from build123d import *

# Parameters (mm, degrees)
BOSS_EXTRUDE1_DEPTH = 1
BOSS_EXTRUDE2_START = 1
BOSS_EXTRUDE2_DEPTH = 1
CUT_EXTRUDE1_REACH  = 128.037
CUT_EXTRUDE2_REACH  = 126.851
SKETCH4_R           = 1.25
CHAMFER1_SIZE       = 1.5
SKETCH5_W           = 55.9
SKETCH5_H           = 5
BOSS_EXTRUDE3_DEPTH = 1.5
CHAMFER3_SIZE       = 0.5


with BuildPart() as part:
    # Sketch1 → Boss-Extrude1 (new body)
    with BuildSketch(Plane.XY):
        with BuildLine():
            Line((67.3, -33.7), (112.5, -33.7))
            Line((112.5, -33.7), (120.2, -33.7))
            Line((120.2, -33.7), (120.2, 33.7))
            Line((120.2, 33.7), (112.5, 33.7))
            Line((112.5, 33.7), (67.3, 33.7))
            ThreePointArc((67.3, 33.7), (66.097918472, 33.202081528), (65.6, 32))
            Line((65.6, 32), (65.6, 6.5))
            ThreePointArc((65.6, 6.5), (64.926345597, 4.873654403), (63.3, 4.2))
            Line((63.3, 4.2), (62, 4.2))
            ThreePointArc((62, 4.2), (60.797918472, 3.702081528), (60.3, 2.5))
            Line((60.3, 2.5), (60.3, -2.5))
            ThreePointArc((60.3, -2.5), (60.797918472, -3.702081528), (62, -4.2))
            Line((62, -4.2), (63.3, -4.2))
            ThreePointArc((63.3, -4.2), (64.926345597, -4.873654403), (65.6, -6.5))
            Line((65.6, -6.5), (65.6, -32))
            ThreePointArc((65.6, -32), (66.097918472, -33.202081528), (67.3, -33.7))
        make_face()
    extrude(amount=BOSS_EXTRUDE1_DEPTH)

    # Sketch2 → Boss-Extrude2 (add)
    with BuildSketch(Plane(origin=(0, 0, 0), x_dir=(-1, 0, 0), z_dir=(0, 0, -1)).offset(BOSS_EXTRUDE2_START)):
        with BuildLine():
            Line((-67.3, 33.7), (-120.2, 33.7))
            Line((-120.2, 33.7), (-120.2, -33.7))
            Line((-120.2, -33.7), (-67.3, -33.7))
            ThreePointArc((-67.3, -33.7), (-66.097918472, -33.202081528), (-65.6, -32))
            Line((-65.6, -32), (-65.6, -6.5))
            ThreePointArc((-65.6, -6.5), (-64.926345597, -4.873654403), (-63.3, -4.2))
            Line((-63.3, -4.2), (-62, -4.2))
            ThreePointArc((-62, -4.2), (-60.797918472, -3.702081528), (-60.3, -2.5))
            Line((-60.3, -2.5), (-60.3, 2.5))
            ThreePointArc((-60.3, 2.5), (-60.797918472, 3.702081528), (-62, 4.2))
            Line((-62, 4.2), (-63.3, 4.2))
            ThreePointArc((-63.3, 4.2), (-64.926345597, 4.873654403), (-65.6, 6.5))
            Line((-65.6, 6.5), (-65.6, 32))
            ThreePointArc((-65.6, 32), (-66.097918472, 33.202081528), (-67.3, 33.7))
        make_face()
        with BuildLine():
            Line((-67.3, 32.7), (-119.2, 32.7))
            Line((-119.2, 32.7), (-119.2, -32.7))
            Line((-119.2, -32.7), (-67.3, -32.7))
            ThreePointArc((-67.3, -32.7), (-66.805025253, -32.494974747), (-66.6, -32))
            Line((-66.6, -32), (-66.6, -6.5))
            Line((-66.6, -6.5), (-66.6, 6.5))
            Line((-66.6, 6.5), (-66.6, 32))
            ThreePointArc((-66.6, 32), (-66.805025253, 32.494974747), (-67.3, 32.7))
        make_face(mode=Mode.SUBTRACT)
    extrude(amount=-BOSS_EXTRUDE2_DEPTH)

    # Cut-Extrude1: up to this face of the body (flat: up to its plane)
    cut_extrude1_end = Plane(part.part.faces().sort_by_distance((62.65, -4.2, 0))[0])
    # Sketch3 → Cut-Extrude1 (cut, up to the picked face)
    with BuildSketch(Plane(origin=(0, 4.2, 0), x_dir=(1, 0, 0), z_dir=(0, 1, 0)), mode=Mode.PRIVATE) as cut_extrude1_sk1:
        Polygon((62, 1), (60.3, -1), (60.3, 1), align=None)
    cut_extrude1_tool1 = split(extrude(cut_extrude1_sk1.sketch, amount=-CUT_EXTRUDE1_REACH, mode=Mode.PRIVATE), bisect_by=cut_extrude1_end, keep=Keep.BOTH, mode=Mode.PRIVATE)
    add(cut_extrude1_tool1.solids().sort_by(Axis((60.866667, 4.2, -0.333333), (0, -1, 0)))[0], mode=Mode.SUBTRACT)

    # Sketch4 → Cut-Extrude2 (cut, up to next)
    with BuildSketch(Plane(origin=(0, 0, -1), x_dir=(-1, 0, 0), z_dir=(0, 0, -1)), mode=Mode.PRIVATE) as cut_extrude2_sk1:
        with Locations((-63.75, 0)):
            Circle(SKETCH4_R)
    cut_extrude2_tool1 = extrude(cut_extrude2_sk1.sketch, amount=-CUT_EXTRUDE2_REACH, mode=Mode.PRIVATE) & part.part
    add(cut_extrude2_tool1.solids().sort_by_distance((63.75, 0, -1))[0], mode=Mode.SUBTRACT)

    # Chamfer1
    chamfer1_edges = [part.edges().sort_by_distance(p)[0] for p in [
        (65, 0, 1),
    ]]
    chamfer(chamfer1_edges, length=CHAMFER1_SIZE)

    # Sketch5 → Boss-Extrude3 (add)
    with BuildSketch(Plane(origin=(0, 0, 0), x_dir=(-1, 0, 0), z_dir=(0, 0, -1))):
        with Locations((-94.55, -22.2)):
            Rectangle(SKETCH5_W, SKETCH5_H)
        with Locations((-94.55, 22.2)):
            Rectangle(SKETCH5_W, SKETCH5_H)
    extrude(amount=BOSS_EXTRUDE3_DEPTH)

    # Chamfer3
    chamfer3_edges = [part.edges().sort_by_distance(p)[0] for p in [
        (122.5, 22.2, -1.5),
        (122.5, -22.2, -1.5),
        (66.6, -22.2, -1.5),
        (66.6, 22.2, -1.5),
    ]]
    chamfer(chamfer3_edges, length=CHAMFER3_SIZE - 0.0001)  # a hair under: the kernel refuses the full size


solid = part.part
The listing builds one solid part. Answer for the finished solid, in the listing's coordinates (mm). A direction names the side the tool comes from. Give positions to 0.01 mm unless a question says otherwise; leave off trailing zeros. Write each loop counter-clockwise with the first axis right and the second up, starting at its lowest first coordinate (ties: lowest second). Pieces come first, ordered by that corner, then holes. Notation, with made-up numbers: (83, -2) -> (124, -2) arc R27 cw to (124, 27) -> close; hole circle Ø9 at (-38, 5.25). An arc over 180 degrees is marked (long way). Use a Markdown table: item, result.
(1) Section C-C, the plane x = 113 is taken. Determine the outline of the cut face in (y, z), then the cut area to 3 significant figures.
Return value:
| item | result |
|---|---|
| outline | (-33.7, -1) -> (-32.7, -1) -> (-32.7, 0) -> (-24.7, 0) -> (-24.7, -1.5) -> (-19.7, -1.5) -> (-19.7, 0) -> (19.7, 0) -> (19.7, -1.5) -> (24.7, -1.5) -> (24.7, 0) -> (32.7, 0) -> (32.7, -1) -> (33.7, -1) -> (33.7, 1) -> (-33.7, 1) -> close |
| area | 84.4 mm2 |
(2) Flat-ended cylindrical pins translate along their axes: P1, Ø0.7, axis at x = 121, y = -22.5, coming from the +Z side; P2, Ø0.8, axis at y = -1, z = -0.5, coming from the -X side (3 decimals); P3, Ø1, axis at x = 63, z = 0.5, coming from the +Y side. Find the tip coordinate at first contact, or state that the pin passes through.
Return value:
| item | result |
|---|---|
| P1 | z = 0 |
| P2 | x = 61.235 |
| P3 | y = 4.21 |
(3) Find the intervals of material crossed by probe 1 along Y at (x, z) = (76, -0.65); probe 2 along Z at (x, y) = (86, -16.5); probe 3 along Y at (x, z) = (63.75, -0.7), in increasing order. Write a range as from..to.
Return value:
| item | result |
|---|---|
| probe 1 | -33.7..-32.7, -24.7..-19.7, 19.7..24.7, 32.7..33.7 |
| probe 2 | 0..1 |
| probe 3 | -4.24..-1.25, 1.25..4.24 |
(4) Determine the mould class of faces 1 (the cylindrical face through (64.94, -4.89, -0.01)), 2 (the flat face through (95, -24.7, -1)), 3 (the flat face through (94, -33.7, 0)) for opening direction X: released by +X, released by -X, zero draft, split by the parting line, or undercut.
Return value:
| item | result |
|---|---|
| face 1 | released by -X |
| face 2 | undercut |
| face 3 | zero draft |
(5) For faces 4 (the flat face through (65.6, 19, 0)), 5 (the flat face through (95, -19.7, -1)), 6 (the flat face through (121, 22, 0)), determine the directions among +Z, -Z, +X, -X, +Y, -Y from which every point of the face is accessible in a straight line to the end or side of a thin tool.
Return value:
| item | result |
|---|---|
| face 4 | +Z, -Z, -X, +Y |
| face 5 | -Z |
| face 6 | +Z, +X, +Y, -Y |
(6) Section A-A, the plane y = 0 is taken. Determine the outline of the cut face in (x, z).
Return value:
| item | result |
|---|---|
| outline | (60.3, 1) -> (62, -1) -> (62.5, -1) -> (62.5, -0.5) -> (61, 1) -> close; (65, -1) -> (66.6, -1) -> (66.6, 0) -> (119.2, 0) -> (119.2, -1) -> (120.2, -1) -> (120.2, 1) -> (66.5, 1) -> (65, -0.5) -> close |
(7) Section D-D, the plane z = 0.45 is taken. Determine the outline of the cut face in (x, y), then the cut area to 3 significant figures.
Return value:
| item | result |
|---|---|
| outline | (60.77, -3.67) arc R1.7 ccw to (62, -4.2) -> (63.3, -4.2) arc R2.3 cw to (65.6, -6.5) -> (65.6, -32) arc R1.7 ccw to (67.3, -33.7) -> (120.2, -33.7) -> (120.2, 33.7) -> (67.3, 33.7) arc R1.7 ccw to (65.6, 32) -> (65.6, 6.5) arc R2.3 cw to (63.3, 4.2) -> (62, 4.2) arc R1.7 ccw to (60.77, 3.67) -> close; hole circle Ø4.4 at (63.75, 0) |
| area | 3,710 mm2 |
